```python
from build123d import *

# Parameters (mm, degrees)
BASPROSKE_W        = 5
BASPROSKE_H        = 6
TOOTHCUT_DEPTH     = 10.848857802
TEETHCUTS_COUNT    = 10
TEETHCUTS_ANGLE    = 324
BORSKE_R           = 1.5
BORE_DEPTH         = 50.0000508
KEYSKE_W           = 1.2
KEYSKE_H           = 2
KEYWAY_DEPTH       = 50.0000508
SKETCH1_W          = 3.96875
SKETCH1_H          = 3.96875
CUT_EXTRUDE1_DEPTH = 10.693816982


with BuildPart() as part:
    # BasProSke → Base-Revolve (revolve)
    with BuildSketch(Plane(origin=(0, 0, 0), x_dir=(1, 0, 0), z_dir=(0, 1, 0)), mode=Mode.PRIVATE) as base_revolve_sk:
        with Locations((2.5, 3)):
            Rectangle(BASPROSKE_W, BASPROSKE_H)
    revolve(base_revolve_sk.sketch.rotate(Axis((-10, 0, 0), (1, 0, 0)), 180), axis=Axis((-10, 0, 0), (1, 0, 0)))

    # TooCutSke → ToothCut (cut, through all)
    with BuildSketch(Plane(origin=(0, 0, 0), x_dir=(0, 0, -1), z_dir=(1, 0, 0))):
        with BuildLine():
            ThreePointArc((0.59278292, 3.701838653), (0, 3.749), (-0.59278292, 3.701838653))
            ThreePointArc((-0.59278292, 3.701838653), (-0.846593509, 4.924114224), (-1.775771316, 5.757784417))
            ThreePointArc((-1.775771316, 5.757784417), (0, 6.0254), (1.775771316, 5.757784417))
            ThreePointArc((1.775771316, 5.757784417), (0.846593509, 4.924114224), (0.59278292, 3.701838653))
        make_face()
    toothcut = extrude(amount=TOOTHCUT_DEPTH, mode=Mode.SUBTRACT)

    # TeethCuts: ToothCut ×10 about axis
    teethcuts_axis = Axis((-10, 0, 0), (1, 0, 0))
    for i in range(1, TEETHCUTS_COUNT):
        add(toothcut.rotate(teethcuts_axis, i * TEETHCUTS_ANGLE / (TEETHCUTS_COUNT - 1)), mode=Mode.SUBTRACT)

    # BorSke → Bore (cut, symmetric)
    with BuildSketch(Plane(origin=(0, 0, 0), x_dir=(0, 0, -1), z_dir=(1, 0, 0))):
        with Locations(Location((0, 0, 0), (0, 0, 180))):
            Circle(BORSKE_R)
    extrude(amount=BORE_DEPTH, both=True, mode=Mode.SUBTRACT)

    # KeySke → Keyway (cut, symmetric)
    with BuildSketch(Plane(origin=(0, 0, 0), x_dir=(0, 0, -1), z_dir=(1, 0, 0))):
        with Locations((0, 1)):
            Rectangle(KEYSKE_W, KEYSKE_H)
    extrude(amount=KEYWAY_DEPTH, both=True, mode=Mode.SUBTRACT)

    # Sketch1 → Cut-Extrude1 (cut, through all)
    with BuildSketch(Plane.ZY):
        Rectangle(SKETCH1_W, SKETCH1_H)
    extrude(amount=-CUT_EXTRUDE1_DEPTH, mode=Mode.SUBTRACT)


solid = part.part
```
The listing builds one solid part. Answer for the finished solid, in the listing's coordinates (mm). A direction names the side the tool comes from. Coordinates: 2 decimals unless noted, no trailing zeros. Write each loop counter-clockwise with the first axis right and the second up, starting at its lowest first coordinate (ties: lowest second). Pieces come first, ordered by that corner, then holes. Notation, with made-up numbers: (56, -1.75) - (88, -1.75) arc R25 ccw to (88, 10.25) - close; hole circle Ø2 at (-2.5, 62). An arc over 180 degrees is marked (long way). Return JSON: item names as keys, results as strings. Group by question number.
1. A cutting plane is placed at A-A, the plane y = 4.75. Determine the outline of the cut face in (x, z).
2. A cutting plane is placed at C-C, the plane z = -3.5. Determine the outline of the cut face in (x, y).
3. Determine the mould class of faces 1 (the flat face through (5, 2.5, 0.1)), 2 (the cylindrical face through (2.465, -4.923, 0.846)), 3 (the cylindrical face through (2.465, -0.724, -4.909)) for opening direction Z: released by +Z, released by -Z, zero draft, split by the parting line, or undercut.
4. Given pin 1 (1.1 mm diameter, centred on x = 2.5, z = 1, fed in from -Y); pin 2 (1.5 mm diameter, centred on x = 1.5, y = 3, fed in from -Z); pin 3 (3 mm diameter, centred on x = 3.5, y = -1.5, fed in from -Z); pin 4 (2 mm diameter, centred on x = 3, z = 0, fed in from +Y), each flat-ended and moving along its own axis, determine where each tip first touches the part or whether it passes through.
5. Which of the six approach directions +Z, -Z, +X, -X, +Y, -Y give full straight-line access (tool end or side, diameter ignored) to faces 4 (the flat face through (0, 2.5, 0.1)), 5 (the flat face through (3, 2, 0))?
6. A cutting plane is placed at B-B, the plane z = 1.25. Determine the outline of the cut face in (x, y).
7. A cutting plane is placed at D-D, the plane z = 4. Determine the outline of the cut face in (x, y), plus the area to 3 significant figures.
8. Straight lines are drawn through the part: L1, parallel to Z at x = 4.35, y = 4.75; L2, parallel to Y at x = 2.95, z = 4.5; L3, parallel to Y at x = 1.95, z = 4. For each, find the intervals that lie inside material, in ascending order.
Ans:
{
 "1": {"outline": "(0, -2.22) - (5, -2.22) - (5, -0.76) - (0, -0.76) - close; (0, 0.76) - (5, 0.76) - (5, 2.22) - (0, 2.22) - close"},
 "2": {"outline": "(0, -3.45) - (5, -3.45) - (5, -1.75) - (0, -1.75) - close; (0, -1.34) - (5, -1.34) - (5, 1.34) - (0, 1.34) - close; (0, 1.75) - (5, 1.75) - (5, 3.45) - (0, 3.45) - close"},
 "3": {"face 1": "zero draft", "face 2": "undercut", "face 3": "undercut"},
 "4": {"pin 1": "y = -5.64", "pin 2": "z = -4.92", "pin 3": "z = -6", "pin 4": "y = 5.15"},
 "5": {"face 4": "+Z, -Z, -X, +Y, -Y", "face 5": "+X, -X"},
 "6": {"outline": "(0, -5.42) - (5, -5.42) - (5, -1.98) - (0, -1.98) - close; (0, 1.98) - (5, 1.98) - (5, 5.42) - (0, 5.42) - close"},
 "7": {"outline": "(0, -3.62) - (5, -3.62) - (5, -1.97) - (0, -1.97) - close; (0, -0.69) - (5, -0.69) - (5, 0.69) - (0, 0.69) - close; (0, 1.97) - (5, 1.97) - (5, 3.62) - (0, 3.62) - close", "area": "23.4 mm²"},
 "8": {"L1": "-2.22 to -0.76, 0.76 to 2.22", "L2": "-3.66 to -2.42, -0.76 to 0.76, 2.42 to 3.66", "L3": "-3.62 to -1.97, -0.69 to 0.69, 1.97 to 3.62"}
}
